Design review of the part shown in the three views and the two pictorial views. Dimensions are in mm from the part's minimum x, y and z. A direction names the side the tool comes from. Round coordinates to 2 decimals unless told otherwise and drop trailing zeros. Loops run counter-clockwise (first coordinate to the right, second up) from the corner with the lowest first, then second, coordinate; pieces in that order, holes last. Notation, with made-up numbers: M 26,80 L 73,80 A17 ccw 73,107 Z; hole C 41,5.25 d6. An arc over 180 degrees is marked long. Return JSON: item names as keys, results as strings. Group by question number.
Q1. For the marked faces 1 and 2, list the 3-axis set-ups (+Z, -Z, +X, -X, +Y, -Y) from which the entire face can be reached by the end or side of a thin tool; tool diameter is ignored.
Q2. Clearance check with flat-ended pins moving along their axes: pin 1 Ø1 at (y, z) = (4.5, 2) entering from -X; pin 2 Ø1 at (x, z) = (2, 1) entering from -Y. State where each tip first meets the part, or that it passes through.
Q3. Consider section A-A (x = 1.6). State the section outline as (y, z) points, and give its area (3 significant figures).
Q4. Consider section C-C (y = 5). State the section outline as (x, z) points.
Q5. Consider section B-B (y = 1). State the section outline as (x, z) points.
Q6. To check wall thickness, follow line 1 along Y through (x, z) = (0.5, 2.35); line 2 along X through (y, z) = (6.5, 1.55); line 3 along X through (y, z) = (3.5, 0.9). State the ranges of each line that lie inside material, in increasing order.
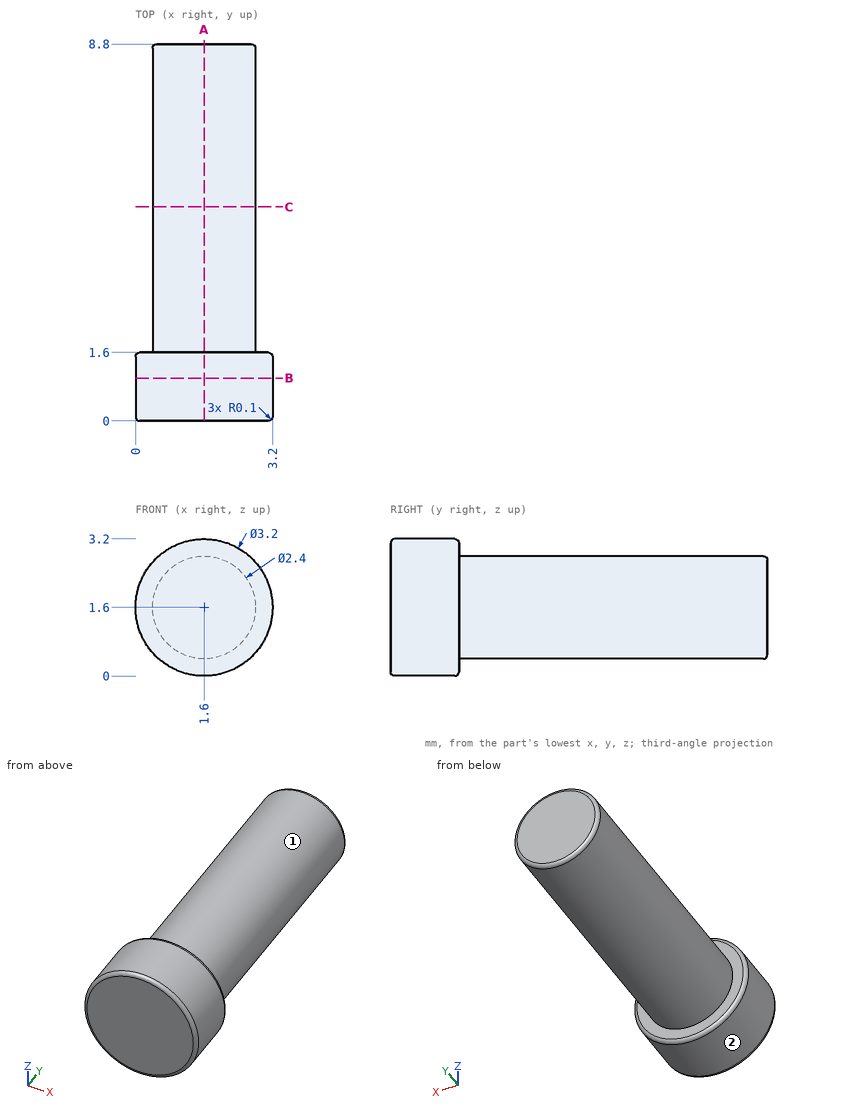
Values:
{
 "1": {"face 1": "+Y", "face 2": "+Y, -Y"},
 "2": {"pin 1": "stops at x = 0.4", "pin 2": "stops at y = 0"},
 "3": {"outline": "M 0,0.1 A0.1 ccw 0.1,0 L 1.5,0 A0.1 ccw 1.6,0.1 L 1.6,0.4 L 8.7,0.4 A0.1 ccw 8.8,0.5 L 8.8,2.7 A0.1 ccw 8.7,2.8 L 1.6,2.8 L 1.6,3.1 A0.1 ccw 1.5,3.2 L 0.1,3.2 A0.1 ccw 0,3.1 Z", "area": "22.4 mm2"},
 "4": {"outline": "C 1.6,1.6 d2.4"},
 "5": {"outline": "C 1.6,1.6 d3.2"},
 "6": {"line 1": "y = 0 to 1.6", "line 2": "x = 0.4 to 2.8", "line 3": "x = 0.63 to 2.57"}
}
